```python
from build123d import *

# Parameters (mm, degrees)
BOX003_W          = 0.5
BOX003_H          = 5
BOX003_DEPTH      = 0.5
BOX001_W          = 5
BOX001_H          = 5
BOX001_DEPTH      = 7.8
BOX002_W          = 0.5
BOX002_H          = 5
BOX002_DEPTH      = 0.5
BOX_W             = 4
BOX_H             = 3
BOX_DEPTH         = 2
BOX_ROLL_ANGLE    = -45
CYLINDER001_R     = 0.3
CYLINDER001_DEPTH = 11
CYLINDER_R        = 2
CYLINDER_DEPTH    = 8
CYLINDER002_R     = 0.5
CYLINDER002_DEPTH = 2
PAD_DEPTH         = 2


with BuildPart() as obj1:
    # Box003 → Box003 (new body)
    with BuildSketch(Plane(origin=(1, -3.5, -0.5), x_dir=(1, 0, 0), z_dir=(0, 0, 1))):
        with Locations((0.25, 2.5)):
            Rectangle(BOX003_W, BOX003_H)
    extrude(amount=BOX003_DEPTH)


with BuildPart() as obj2:
    # Box001 → Box001 (new body)
    with BuildSketch(Plane(origin=(-2.5, -2.5, 0), x_dir=(1, 0, 0), z_dir=(0, 0, 1))):
        with Locations((2.5, 2.5)):
            Rectangle(BOX001_W, BOX001_H)
    extrude(amount=BOX001_DEPTH)


with BuildPart() as obj3:
    # Box002 → Box002 (new body)
    with BuildSketch(Plane(origin=(-1.5, -3.5, -0.5), x_dir=(1, 0, 0), z_dir=(0, 0, 1))):
        with Locations((0.25, 2.5)):
            Rectangle(BOX002_W, BOX002_H)
    extrude(amount=BOX002_DEPTH)


with BuildPart() as obj4:
    # Box → Box (new body)
    with BuildSketch(Plane.XY):
        with Locations((2, 1.5)):
            Rectangle(BOX_W, BOX_H)
    extrude(amount=BOX_DEPTH)


with BuildPart() as obj4_1:
    # Box roll: moved
    add(obj4.part.rotate(Axis((0, 0, 0), (1, 0, 0)), BOX_ROLL_ANGLE))


with BuildPart() as obj4_2:
    # Box placement: moved
    add(obj4_1.part.moved(Location((-1, 0, 11))))


with BuildPart() as achse:
    # Cylinder001 → Cylinder001 (new body)
    with BuildSketch(Plane.XY):
        Circle(CYLINDER001_R)
    extrude(amount=CYLINDER001_DEPTH)


with BuildPart() as motor:
    # Cylinder → Cylinder (new body)
    with BuildSketch(Plane.XY):
        Circle(CYLINDER_R)
    extrude(amount=CYLINDER_DEPTH)


with BuildPart() as zylinder:
    # Cylinder002 → Cylinder002 (new body)
    with BuildSketch(Plane.XY.offset(9)):
        Circle(CYLINDER002_R)
    extrude(amount=CYLINDER002_DEPTH)


with BuildPart() as motor001:
    # Sketch → Pad (new body)
    with BuildSketch(Plane.XY.offset(9)):
        with BuildLine():
            Line((0, 2), (0, -2))
            ThreePointArc((0, -2), (2, 0), (0, 2))
        make_face()
    extrude(amount=PAD_DEPTH)

    # Fusion: union Achse, Motor, Zylinder
    add(achse.part)
    add(motor.part)
    add(zylinder.part)

    # Cut: cut obj4
    add(obj4_2.part, mode=Mode.SUBTRACT)

    # Fusion001: union obj1, obj2, obj3
    add(obj1.part)
    add(obj2.part)
    add(obj3.part)


solid = motor001.part
```
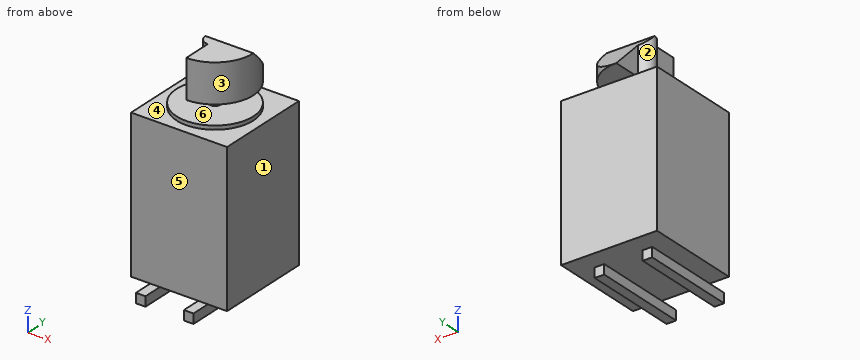
For this review, take the finished solid that the model builds, in its own axes (mm). Face numbers are marked on the shaded views. A direction names the side the tool comes from. Round coordinates to 2 decimals unless told otherwise and drop trailing zeros. Order: outer loops, then holes, each group sorted by start corner. A loop starts at its lowest first (then second) coordinate and runs counter-clockwise, first axis right, second up.
Q1. We need section A-A, the plane x = -1.2. Give the boundary of the cut face in (y, z), plus the area to 3 significant figures.
Findings below:
outline: (-3.5, -0.5) - (1.5, -0.5) - (1.5, 0) - (2.5, 0) - (2.5, 7.8) - (1.6, 7.8) - (1.6, 8) - (-1.6, 8) - (-1.6, 7.8) - (-2.5, 7.8) - (-2.5, 0) - (-3.5, 0) - close
area: 42.1 mm2
Q2. Insertion check: P1, Ø1.6, axis at y = 1, z = 9.5, coming from the -X side; P2, Ø2.5, axis at x = 0, y = 1, coming from the -Z side; P3, Ø1.5, axis at x = 0, z = 2, coming from the -Y side. Each pin has a flat end and moves straight along its axis. Give the tip position at first contact, or say it passes through.
Findings below:
P1: stops at x = -0.46
P2: stops at z = -0.5
P3: stops at y = -2.5
Q3. We need section C-C, the plane y = -2.25. Give the boundary of the cut face in (x, z).
Findings below:
outline: (-2.5, 0) - (-1.5, 0) - (-1.5, -0.5) - (-1, -0.5) - (-1, 0) - (1, 0) - (1, -0.5) - (1.5, -0.5) - (1.5, 0) - (2.5, 0) - (2.5, 7.8) - (-2.5, 7.8) - close
Q4. Mouldability with a two-part tool opening along Z and no side actions: class the marked faces 4, 5 and 6 as pulls with the +Z half, pulls with the -Z half, needs draft (parallel to the pull), parting line crosses it, or undercut.
Findings below:
face 4: pulls with the +Z half
face 5: needs draft
face 6: undercut
Q5. We need section D-D, the plane z = 7.5. Give the boundary of the cut face in (x, y), plus the area to 3 significant figures.
Findings below:
outline: (-2.5, -2.5) - (2.5, -2.5) - (2.5, 2.5) - (-2.5, 2.5) - close
area: 25.0 mm2
Q6. We need section B-B, the plane y = -0.9. Give the boundary of the cut face in (x, z).
Findings below:
outline: (-2.5, 0) - (-1.5, 0) - (-1.5, -0.5) - (-1, -0.5) - (-1, 0) - (1, 0) - (1, -0.5) - (1.5, -0.5) - (1.5, 0) - (2.5, 0) - (2.5, 7.8) - (1.79, 7.8) - (1.79, 8) - (-1.79, 8) - (-1.79, 7.8) - (-2.5, 7.8) - close; (0, 9) - (1.79, 9) - (1.79, 11) - (0, 11) - close
Q7. Machinability: for the marked faces 1, 2 and 3, which of the approach directions +Z, -Z, +X, -X, +Y, -Y give a long, thin tool a straight path to every point of the face, cutting with its end or side? Answer none if there is none.
Findings below:
face 1: +Z, -Z, +X, +Y, -Y
face 2: +Z, -X
face 3: +Z, +X
Q8. Wall thickness on line 1 (Y direction, x = 1.3, z = 3.75); line 2 (Z direction, x = 1.6, y = 0.3); line 3 (Z direction, x = 0.8, y = 0.95): over which ranges is each line inside the solid? List them lowest first.
Findings below:
line 1: y = -2.5 to 2.5
line 2: z = 0 to 8, 9 to 10.7
line 3: z = 0 to 8, 9 to 10.05
